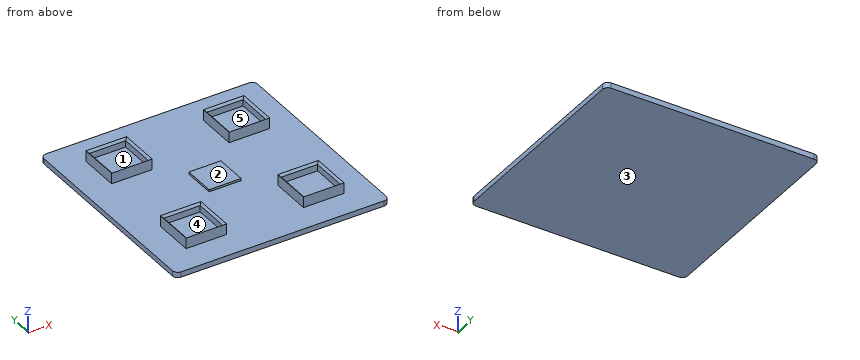
Autodesk Inventor part; units mm, degrees
ref_plane "YZ Plane" through (0, 0, 0) normal (1, 0, 0) x (0, 1, 0)
ref_plane "XZ Plane" through (0, 0, 0) normal (0, 1, 0) x (-1, 0, 0)
ref_plane "XY Plane" through (0, 0, 0) normal (0, 0, 1) x (1, 0, 0)
sketch "Náčrt1" plane through (0, 0, 0) normal (0, 0, 1) x (1, 0, 0)
  line L0 (-140, 0) -> (140, 0)
  line L1 (0, -140) -> (0, 140)
  line L2 (-100, 100) -> (100, 100)
  line L3 (100, 100) -> (100, -100)
  line L4 (100, -100) -> (-100, -100)
  line L5 (-100, -100) -> (-100, 100)
  point P0 (0, 0)
  point P1 (0, 100)
  point P2 (100, 0)
  dimension "d0" = 200
  dimension "d1" = 200
extrude "Vysunutí1" add sketch "Náčrt1" along normal blind 5
fillet "Zaoblení1" radius 5 4 edges at (100, 100, 2.5) (-100, 100, 2.5) (-100, -100, 2.5) (100, -100, 2.5)
sketch "Náčrt2" plane through (0, 0, 5) normal (0, 0, 1) x (1, 0, 0)
  line L0 (-100, 95) -> (-100, -95)
  line L1 (-95, -100) -> (95, -100)
  arc A0 (95, -100) -> (100, -95) centre (95, -95) ccw
  line L2 (100, -95) -> (100, 95)
  arc A1 (100, 95) -> (95, 100) centre (95, 95) ccw
  line L3 (95, 100) -> (-95, 100)
  arc A2 (-95, 100) -> (-100, 95) centre (-95, 95) ccw
  line L4 (-100, 95) -> (-100, -95)
  arc A3 (-100, -95) -> (-95, -100) centre (-95, -95) ccw
  line L5 (-95, -100) -> (95, -100)
  line L6 (-141.4497, 0) -> (141.4497, 0)
  line L7 (0, -141.4497) -> (0, 141.4497)
  line L8 (-15, -15) -> (15, -15)
  line L9 (15, -15) -> (15, 15)
  line L10 (15, 15) -> (-15, 15)
  line L11 (-15, 15) -> (-15, -15)
  line L12 (-72, -72) -> (-38, -72)
  line L13 (-38, -72) -> (-38, -38)
  line L14 (-38, -38) -> (-72, -38)
  line L15 (-72, -38) -> (-72, -72)
  line L16 (-72, 38) -> (-38, 38)
  line L17 (-72, 72) -> (-72, 38)
  line L18 (-38, 72) -> (-72, 72)
  line L19 (-38, 38) -> (-38, 72)
  line L20 (38, -72) -> (72, -72)
  line L21 (38, -38) -> (38, -72)
  line L22 (72, -38) -> (38, -38)
  line L23 (72, -72) -> (72, -38)
  line L24 (38, 38) -> (72, 38)
  line L25 (38, 72) -> (38, 38)
  line L26 (72, 72) -> (38, 72)
  line L27 (72, 38) -> (72, 72)
  point P0 (0, 0)
  point P1 (-15, 0)
  point P2 (0, 15)
  dimension "d5" = 30
  dimension "d6" = 30
  dimension "d8" = 34
  dimension "d9" = 34
  dimension "d10" = 28
  dimension "d11" = 28
  dimension "d14" = 110
  dimension "d17" = 110
extrude "Vysunutí2" add sketch "Náčrt2" along normal blind 2 contours L11 L10 L7 L6 | L6 L7 L8 L11 | L7 L10 L9 L6 | L6 L9 L8 L7 | L15 L14 L13 L12 | L17 L18 L19 L16 | L21 L22 L23 L20 | L25 L26 L27 L24
sketch "Náčrt4" plane through (0, 0, 5) normal (0, 0, 1) x (1, 0, 0)
  line L0 (-38, 38) -> (-72, 38)
  line L1 (-72, 38) -> (-72, 72)
  line L2 (-72, 72) -> (-38, 72)
  line L3 (-38, 72) -> (-38, 38)
  line L4 (72, 38) -> (38, 38)
  line L5 (38, 38) -> (38, 72)
  line L6 (38, 72) -> (72, 72)
  line L7 (72, 72) -> (72, 38)
  line L8 (-15, 15) -> (15, 15)
  line L9 (15, 15) -> (15, -15)
  line L10 (15, -15) -> (-15, -15)
  line L11 (-15, -15) -> (-15, 15)
  line L12 (72, -72) -> (38, -72)
  line L13 (38, -72) -> (38, -38)
  line L14 (38, -38) -> (72, -38)
  line L15 (72, -38) -> (72, -72)
  line L16 (-38, -38) -> (-38, -72)
  line L17 (-38, -72) -> (-72, -72)
  line L18 (-72, -72) -> (-72, -38)
  line L19 (-72, -38) -> (-38, -38)
  arc A0 (95, -100) -> (100, -95) centre (95, -95) ccw
  line L20 (100, -95) -> (100, 95)
  arc A1 (100, 95) -> (95, 100) centre (95, 95) ccw
  line L21 (95, 100) -> (-95, 100)
  arc A2 (-95, 100) -> (-100, 95) centre (-95, 95) ccw
  line L22 (-100, 95) -> (-100, -95)
  arc A3 (-100, -95) -> (-95, -100) centre (-95, -95) ccw
  line L23 (-95, -100) -> (95, -100)
  line L24 (-38, -38) -> (-72, -38)
  line L25 (-72, -38) -> (-72, -72)
  line L26 (-72, -72) -> (-38, -72)
  line L27 (-38, -72) -> (-38, -38)
  line L28 (-15, 15) -> (-15, -15)
  line L29 (-15, -15) -> (15, -15)
  line L30 (15, -15) -> (15, 15)
  line L31 (15, 15) -> (-15, 15)
  line L32 (-38, 72) -> (-72, 72)
  line L33 (-38, 38) -> (-38, 72)
  line L34 (-38, 72) -> (-72, 72)
  line L35 (-72, 72) -> (-72, 38)
  line L36 (-72, 38) -> (-38, 38)
  line L37 (72, 38) -> (72, 72)
  line L38 (72, 72) -> (38, 72)
  line L39 (38, 72) -> (38, 38)
  line L40 (38, 38) -> (72, 38)
  line L41 (72, -72) -> (72, -38)
  line L42 (72, -38) -> (38, -38)
  line L43 (38, -38) -> (38, -72)
  line L44 (38, -72) -> (72, -72)
  line L45 (0, -141.4497) -> (0, 141.4497)
  line L46 (-141.4497, 0) -> (141.4497, 0)
  line L47 (-74, -74) -> (-36, -74)
  line L48 (-36, -74) -> (-36, -36)
  line L49 (-36, -36) -> (-74, -36)
  line L50 (-74, -36) -> (-74, -74)
  line L51 (-36, 36) -> (-36, 74)
  line L52 (-74, 36) -> (-36, 36)
  line L53 (-36, 74) -> (-74, 74)
  line L54 (-74, 74) -> (-74, 36)
  line L55 (74, -74) -> (74, -36)
  line L56 (36, -74) -> (74, -74)
  line L57 (74, -36) -> (36, -36)
  line L58 (36, -36) -> (36, -74)
  line L59 (74, 36) -> (74, 74)
  line L60 (36, 36) -> (74, 36)
  line L61 (74, 74) -> (36, 74)
  line L62 (36, 74) -> (36, 36)
  point P0 (0, 0)
  dimension "d22" = 38
  dimension "d23" = 38
  dimension "d24" = 2
  dimension "d25" = 2
  dimension "d28" = 110
  dimension "d31" = 110
extrude "Vysunutí3" add sketch "Náčrt4" along normal blind 10 contours L50 L49 L48 L47 | L52 L54 L53 L51 | L56 L58 L57 L55 | L60 L62 L61 L59
chamfer "Zkosení1" distance 2 angle 45 16 edges at (-55, -72, 15) (-72, -55, 15) (-55, -38, 15) (-38, -55, 15) (-55, 38, 15) (-72, 55, 15) (-55, 72, 15) (-38, 55, 15) (38, -55, 15) (55, -38, 15) (55, -72, 15) (72, -55, 15) (55, 38, 15) (38, 55, 15) (55, 72, 15) (72, 55, 15)
properties part number "testovaci_podlozka"
Verification items for the finished model (mm, model axes). Face numbers are marked on the shaded views. A direction names the side the tool comes from. Round coordinates to 2 decimals unless told otherwise and drop trailing zeros. Write each loop counter-clockwise with the first axis right and the second up, starting at its lowest first coordinate (ties: lowest second). Pieces come first, ordered by that corner, then holes.
(1) Section check C-C (x = 12). Enter the section's corners in (y, z), plus the area to 3 significant figures.
Returned:
outline: (-100, 0) - (100, 0) - (100, 5) - (15, 5) - (15, 7) - (-15, 7) - (-15, 5) - (-100, 5) - close
area: 1,060 mm2
(2) Depth check by flat-ended pin: pin 1 Ø0.6 at (y, z) = (2, 6) entering from +X; pin 2 Ø12 at (x, y) = (33, 73) entering from +Z; pin 3 Ø17 at (x, y) = (47.5, 49) entering from +Z; pin 4 Ø6.5 at (y, z) = (-58.5, 9.5) entering from +X. Enter the tip coordinate at first touch or a pass-through.
Returned:
pin 1: stops at x = 15
pin 2: stops at z = 15
pin 3: stops at z = 7
pin 4: stops at x = 74
(3) Material ranges on line 1 (X direction, y = -49.5, z = 8); line 2 (X direction, y = -41, z = 6), recorded low to high.
Returned:
line 1: x = -74 to -72, -38 to -36, 36 to 38, 72 to 74
line 2: x = -74 to -36, 36 to 74
(4) Access from +Z, -Z, +X, -X, +Y, -Y to the whole of each face (thin tool, end or side, straight path). Record for the marked faces 1 and 2.
Returned:
face 1: +Z
face 2: +Z, +X, -X, +Y, -Y
(5) Section check D-D (y = -79). Enter the section's corners in (x, z).
Returned:
outline: (-100, 0) - (100, 0) - (100, 5) - (-100, 5) - close
(6) Mould release check, pull along Y, two halves, no side actions. Record for the marked faces 3, 4 and 5: pulls with the +Y half, pulls with the -Y half, needs draft (parallel to the pull), parting line crosses it, or undercut.
Returned:
face 3: needs draft
face 4: undercut
face 5: undercut
